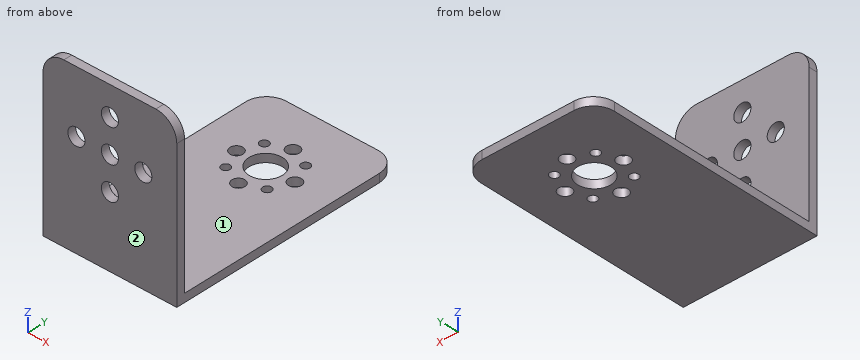
from build123d import *

# Parameters (mm, degrees)
SKETCH_2_W          = 32
SKETCH_2_H          = 40
EXTRUDE_1_DEPTH     = 2
SKETCH_3_W          = 32
SKETCH_3_H          = 2
EXTRUDE_2_DEPTH     = 55
SKETCH_6_R          = 2.05
CUT_EXTRUDE_2_DEPTH = 61.671245248
FILLET_1_R          = 5
SKETCH1_R           = 4
SKETCH1_R_2         = 1.55
SKETCH1_R_3         = 1.05
CUT_EXTRUDE1_DEPTH  = 10


with BuildPart() as part:
    # 草图2 → 凸台-拉伸1 (new body)
    with BuildSketch(Plane(origin=(0, 0, 0), x_dir=(1, 0, 0), z_dir=(0, 1, 0))):
        Rectangle(SKETCH_2_W, SKETCH_2_H)
    extrude(amount=EXTRUDE_1_DEPTH)

    # 草图3 → 凸台-拉伸2 (add)
    with BuildSketch(Plane(origin=(0, 2, 0), x_dir=(1, 0, 0), z_dir=(0, 1, 0))):
        with Locations((0, 19)):
            Rectangle(SKETCH_3_W, SKETCH_3_H)
    extrude(amount=EXTRUDE_2_DEPTH)

    # 草图6 → 切除-拉伸2 (cut, through all)
    with BuildSketch(Plane(origin=(0, 2, 0), x_dir=(1, 0, 0), z_dir=(0, 1, 0))):
        with Locations(Location((0, -5, 0), (0, 0, 270))):
            Circle(SKETCH_6_R)
        with Locations(Location((-8, -5, 0), (0, 0, 270))):
            Circle(SKETCH_6_R)
        with Locations(Location((8, -5, 0), (0, 0, 270))):
            Circle(SKETCH_6_R)
        with Locations(Location((0, 3, 0), (0, 0, 270))):
            Circle(SKETCH_6_R)
        with Locations(Location((0, -13, 0), (0, 0, 270))):
            Circle(SKETCH_6_R)
    extrude(amount=-CUT_EXTRUDE_2_DEPTH, mode=Mode.SUBTRACT)

    # 圆角1
    fillet_1_edges = [part.edges().sort_by_distance(p)[0] for p in [
        (-16, 57, -19),
        (16, 57, -19),
        (16, 1, 20),
        (-16, 1, 20),
    ]]
    fillet(fillet_1_edges, radius=FILLET_1_R)

    # Sketch1 → Cut-Extrude1 (cut)
    with BuildSketch(Plane.XY.offset(-18)):
        with Locations((0, 40)):
            Circle(SKETCH1_R)
        with Locations((0, 47)):
            Circle(SKETCH1_R_2)
        with Locations((4.949747468, 44.949747468)):
            Circle(SKETCH1_R_3)
        with Locations((7, 40)):
            Circle(SKETCH1_R_2)
        with Locations((4.949747468, 35.050252532)):
            Circle(SKETCH1_R_3)
        with Locations((0, 33)):
            Circle(SKETCH1_R_2)
        with Locations((-4.949747468, 35.050252532)):
            Circle(SKETCH1_R_3)
        with Locations((-4.949747468, 44.949747468)):
            Circle(SKETCH1_R_3)
        with Locations((-7, 40)):
            Circle(SKETCH1_R_2)
    extrude(amount=-CUT_EXTRUDE1_DEPTH, mode=Mode.SUBTRACT)


solid = part.part
Here's how the part is built. I have some questions about the finished solid (model axes, mm). Face numbers are marked on the shaded views. A direction names the side the tool comes from. Give positions to 0.01 mm unless a question says otherwise; leave off trailing zeros. Loops run counter-clockwise (first coordinate to the right, second up) from the corner with the lowest first, then second, coordinate; pieces in that order, holes last. Notation, with made-up numbers: (-16, 39) -> (35, 39) arc R23 cw to (35, 54) -> close; hole circle Ø3 at (-30.5, -24.75). An arc over 180 degrees is marked (long way). One line per item, written item: value.
Q1. Suppose I cut it at C-C on y = 33. Please give me the cut outline in (x, z).
Answers follow:
outline: (-16, -20) -> (-1.55, -20) -> (-1.55, -18) -> (-16, -18) -> close; (1.55, -20) -> (16, -20) -> (16, -18) -> (1.55, -18) -> close
Q2. Suppose I cut it at A-A on x = 0. State how many separate pieces and enclosed holes the cut face has, then the cut area to 3 significant figures.
Answers follow:
separate pieces: 7
enclosed holes: 0
area: 137 mm^2
Q3. If I drill on line 1 along X through (y, z) = (1.05, 5); line 2 along Y through (x, z) = (0, -18.65); line 3 along Y through (x, z) = (-6, 7), over which ranges is the centre line in solid material (lowest first)?
Answers follow:
line 1: -16 to -10.05, -5.95 to -2.05, 2.05 to 5.95, 10.05 to 16
line 2: 0 to 31.45, 34.55 to 36, 44 to 45.45, 48.55 to 57
line 3: 0 to 2
Q4. Suppose I cut it at B-B on z = 13. Please give me the cut outline in (x, y), then the cut area to 3 significant figures.
Answers follow:
outline: (-16, 0) -> (-2.05, 0) -> (-2.05, 2) -> (-16, 2) -> close; (2.05, 0) -> (16, 0) -> (16, 2) -> (2.05, 2) -> close
area: 55.8 mm^2
Q5. On a 3-axis mill with a long thin cutter (end or side, diameter ignored), from which of +Z, -Z, +X, -X, +Y, -Y can I reach the whole of each face in a straight line? I mean the marked faces 1 and 2. Say none if no direction works.
Answers follow:
face 1: +Z, +X, -X, +Y
face 2: +Z, -Z, +X, -X, -Y
Q6. Suppose I cut it at D-D on z = 5. Please give me the cut outline in (x, y).
Answers follow:
outline: (-16, 0) -> (-10.05, 0) -> (-10.05, 2) -> (-16, 2) -> close; (-5.95, 0) -> (-2.05, 0) -> (-2.05, 2) -> (-5.95, 2) -> close; (2.05, 0) -> (5.95, 0) -> (5.95, 2) -> (2.05, 2) -> close; (10.05, 0) -> (16, 0) -> (16, 2) -> (10.05, 2) -> close
Q7. I'm going to push flat-ended pins straight in: pin 1 Ø8 at (x, y) = (-5.5, 8.5) entering from +Z; pin 2 Ø2.5 at (x, y) = (-4.95, 44.95) entering from -Z; pin 3 Ø2.5 at (x, z) = (0, 5) entering from +Y; pin 4 Ø1 at (x, z) = (0, -13) entering from +Y. Where does each tip first touch, or does it pass through?
Answers follow:
pin 1: z = -18
pin 2: z = -20
pin 3: through
pin 4: y = 2
